Autodesk Inventor part; units mm, degrees
ref_plane "YZ Plane" through (0, 0, 0) normal (1, 0, 0) x (0, 1, 0)
ref_plane "XZ Plane" through (0, 0, 0) normal (0, 1, 0) x (-1, 0, 0)
ref_plane "XY Plane" through (0, 0, 0) normal (0, 0, 1) x (1, 0, 0)
sketch "Skizze1" plane through (0, 0, 0) normal (0, 1, 0) x (-1, 0, 0)
  circle A0 centre (0, 0) radius 9.5
  dimension "d0" = 19
extrude "Extrusion1" add sketch "Skizze1" along normal blind 16.5
sketch "Skizze2" plane through (0, 16.5, 0) normal (0, 1, 0) x (1, 0, 0)
  circle A0 centre (0, 0) radius 8
  dimension "d3" = 16
extrude "Extrusion2" cut sketch "Skizze2" against normal blind 15
sketch "Skizze3" plane through (0, 0, 0) normal (0, -1, 0) x (1, 0, 0)
  circle A0 centre (0, 0) radius 9.5
hole "Bohrung1" at (0, 0, 0) direction (0, 1, 0) diameter 2.459 depth 1.5
properties part number "23"
Check sheet for the modelled part. Datum: model origin and axes. Units: mm. A direction names the side the tool comes from. Coordinates: 2 decimals unless noted, no trailing zeros. Write each loop counter-clockwise with the first axis right and the second up, starting at its lowest first coordinate (ties: lowest second). Pieces come first, ordered by that corner, then holes. Notation, with made-up numbers: M 61,74 L 81,74 A18 ccw 81,80 Z; hole C 67,21.25 d7. An arc over 180 degrees is marked long. Use one line per item in the form item = value.
Item 1: Gauge pin test, flat ends, axial feed: pin 1 Ø2 at (x, z) = (2, -5) entering from +Y; pin 2 Ø4 at (y, z) = (14.5, -2.5) entering from +X. Record the tip position at first contact, or that the pin passes through.
Answer below:
pin_1 = 1.5
pin_2 = 9.49
Item 2: Sectioned sample at C-C, the plane y = 1. Record the cut outline in (x, z), and give its area (3 significant figures).
Answer below:
outline = C 0,0 d19; hole C 0,0 d2.46
area = 279 mm^2
Item 3: Material ranges on L1, parallel to Z at x = 0, y = 0.85; L2, parallel to Y at x = -1.5, z = 0.25; L3, parallel to Z at x = 0, y = 9.25, recorded low to high. Write a range as from..to.
Answer below:
L1 = -9.5..-1.23, 1.23..9.5
L2 = 0..1.5
L3 = -9.5..-8, 8..9.5
Item 4: Release check for a two-part mould opening along X. For faces 3 (the face through (0.748, 0.76, 0.976)), 4 (the face through (-1.73, 9.1, 7.81)), 5 (the face through (-4.38, 8.13, 8.43)), 6 (the face through (0, 0, -2)) record: pulls with the +X half, pulls with the -X half, needs draft (parallel to the pull), parting line crosses it, or undercut.
Answer below:
face_3 = undercut
face_4 = undercut
face_5 = parting line crosses it
face_6 = needs draft
Item 5: Sectioned sample at A-A, the plane x = 0. Record the cut outline in (y, z).
Answer below:
outline = M 0,-9.5 L 16.5,-9.5 L 16.5,-8 L 1.5,-8 L 1.5,-1.23 L 0,-1.23 Z; M 0,1.23 L 1.5,1.23 L 1.5,8 L 16.5,8 L 16.5,9.5 L 0,9.5 Z
Item 6: Sectioned sample at D-D, the plane z = -4. Record the cut outline in (x, y), and give its area (3 significant figures).
Answer below:
outline = M -8.62,0 L 8.62,0 L 8.62,16.5 L 6.93,16.5 L 6.93,1.5 L -6.93,1.5 L -6.93,16.5 L -8.62,16.5 Z
area = 76.5 mm^2
Item 7: Set-up check for faces 1 (the face through (4.3, 16.5, -7)), 2 (the face through (0, 1.5, 2)): record each of +Z, -Z, +X, -X, +Y, -Y from which the full face is reachable in a straight line by a thin tool's end or side.
Answer below:
face_1 = +Z, -Z, +X, -X, +Y
face_2 = +Y
Item 8: Sectioned sample at B-B, the plane z = 0. Record the cut outline in (x, y).
Answer below:
outline = M -9.5,0 L -1.23,0 L -1.23,1.5 L -8,1.5 L -8,16.5 L -9.5,16.5 Z; M 1.23,0 L 9.5,0 L 9.5,16.5 L 8,16.5 L 8,1.5 L 1.23,1.5 Z
